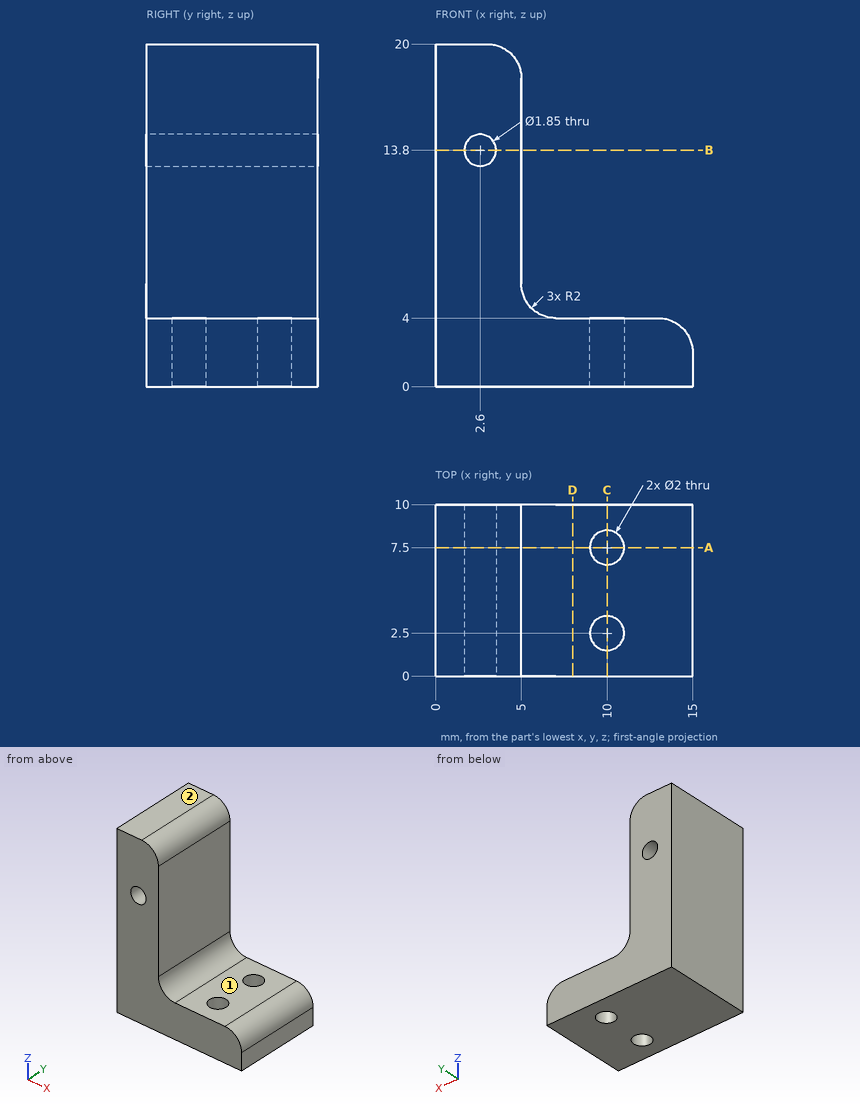
Geometry: see drawing. Coordinates: mm, zero at the bounding-box minimum. A direction names the side the tool comes from. Give positions to 0.01 mm unless a question says otherwise; leave off trailing zeros. Loops run counter-clockwise (first coordinate to the right, second up) from the corner with the lowest first, then second, coordinate; pieces in that order, holes last. Notation, with made-up numbers: (-22.75, 68) -> (-8.75, 68) arc R19 ccw to (-8.75, 89) -> close; hole circle Ø11 at (-1.75, 22). An arc over 180 degrees is marked (long way). Answer as a JSON object with one key per item and string values. Group by question number.
Item 1: Cut plane D-D, the plane x = 8. Return the cut outline in (y, z).
Item 2: Line query: probe 1 along Y at (x, z) = (10, 1.45); probe 2 along X at (y, z) = (6.5, 13.8) (3 decimals); probe 3 along Z at (x, y) = (8.5, 5.5). Output: solid intervals per line, ascending.
Item 3: Cut plane C-C, the plane x = 10. Return the cut outline in (y, z).
Item 4: Cut plane A-A, the plane y = 7.5. Return the cut outline in (x, z) (3 decimals).
Item 5: Pin query (flat end, axial travel): P1, Ø5, axis at y = 4.5, z = 9.5, coming from the +X side; P2, Ø1.7, axis at x = 2.6, z = 13.8, coming from the -Y side; P3, Ø3, axis at x = 10.5, y = 5, coming from the +Z side. Return the tip coordinate at first contact, or that it passes through.
Item 6: Reachability of the marked faces 1 and 2 from +Z, -Z, +X, -X, +Y, -Y: full face, straight path, thin tool, end or side. Return the list, or none.
Item 7: Cut plane B-B, the plane z = 13.8. Return the cut outline in (x, y) (3 decimals).
Checks:
{
 "1": {"outline": "(0, 0) -> (10, 0) -> (10, 4) -> (0, 4) -> close"},
 "2": {"probe 1": "y = 0 to 1.5, 3.5 to 6.5, 8.5 to 10", "probe 2": "x = 0 to 1.675, 3.525 to 5", "probe 3": "z = 0 to 4"},
 "3": {"outline": "(0, 0) -> (1.5, 0) -> (1.5, 4) -> (0, 4) -> close; (3.5, 0) -> (6.5, 0) -> (6.5, 4) -> (3.5, 4) -> close; (8.5, 0) -> (10, 0) -> (10, 4) -> (8.5, 4) -> close"},
 "4": {"outline": "(0, 0) -> (9, 0) -> (9, 4) -> (7, 4) arc R2 cw to (5, 6) -> (5, 18) arc R2 ccw to (3, 20) -> (0, 20) -> close; (11, 0) -> (15, 0) -> (15, 2) arc R2 ccw to (13, 4) -> (11, 4) -> close; hole circle Ø1.85 at (2.6, 13.8)"},
 "5": {"P1": "stops at x = 5", "P2": "passes through", "P3": "stops at z = 4"},
 "6": {"face 1": "+Z, +X, +Y, -Y", "face 2": "+Z, +X, -X, +Y, -Y"},
 "7": {"outline": "(0, 0) -> (1.675, 0) -> (1.675, 10) -> (0, 10) -> close; (3.525, 0) -> (5, 0) -> (5, 10) -> (3.525, 10) -> close"}
}
